Here's the drawing with two shaded views (mm, measured from the low corner). I have some questions. Round coordinates to 2 decimals unless told otherwise and drop trailing zeros. Write each loop counter-clockwise with the first axis right and the second up, starting at its lowest first coordinate (ties: lowest second). Pieces come first, ordered by that corner, then holes. Notation, with made-up numbers: M 8,-29.5 L 22,-29.5 A34 cw 22,8.5 Z; hole C -32.75,17 d10. An arc over 180 degrees is marked long. Answer as a JSON object with one key per item and string values. Group by question number.
1) I'm going to push flat-ended pins straight in: pin 1 Ø2 at (x, z) = (46, 46) entering from -Y; pin 2 Ø3 at (y, z) = (49, 26) entering from -X; pin 3 Ø12 at (x, y) = (67, 35) entering from +Z. Where does each tip first touch, or does it pass through?
2) Suppose I cut it at A-A, the plane x = 50. Write out the boundary of the cut face in (y, z), and give its area (3 significant figures).
3) Suppose I cut it at B-B, the plane y = 48. Write out the boundary of the cut face in (x, z).
4) Suppose I cut it at C-C, the plane z = 24. Write out the boundary of the cut face in (x, y).
5) Suppose I cut it at D-D, the plane x = 92. Write out the boundary of the cut face in (y, z), and give its area (3 significant figures).
6) Please list where these lines run through material, in increasing order: L1, parallel to Z at x = 48.5, y = 43; L2, parallel to Z at x = 50, y = 57; L3, parallel to Y at x = 64, z = 27. Write a range as [from, to].
7) If we mould it in two halves opening along X, with no side actions, what happens to the marked faces 1, 2, 3 and 4? For each: +X half, -X half, draft (parallel to the pull), parting line (faces both ways), or undercut.
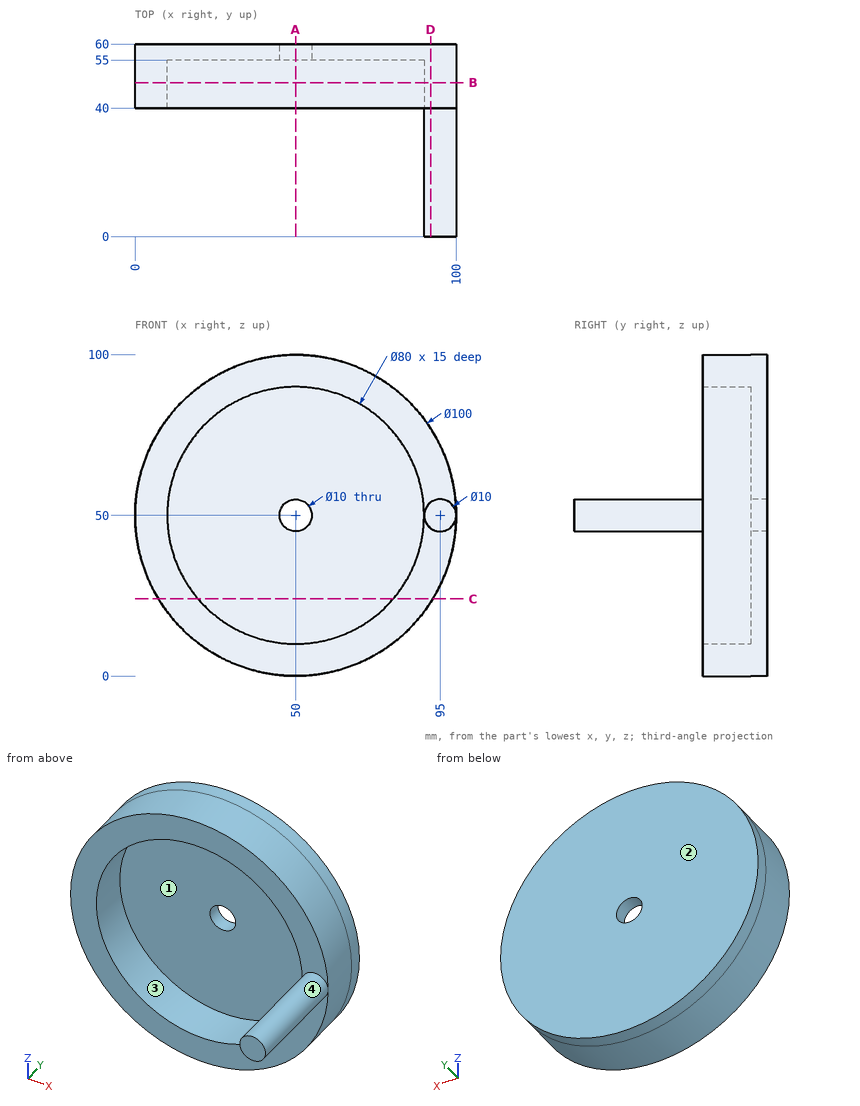
Results:
{
 "1": {"pin 1": "y = 55", "pin 2": "x = 5.35", "pin 3": "z = 98.09"},
 "2": {"outline": "M 40,0 L 60,0 L 60,45 L 55,45 L 55,10 L 40,10 Z; M 40,90 L 55,90 L 55,55 L 60,55 L 60,100 L 40,100 Z", "area": "750 mm^2"},
 "3": {"outline": "C 50,50 d100; hole C 50,50 d80"},
 "4": {"outline": "M 7.29,40 L 19.6,40 L 19.6,55 L 80.4,55 L 80.4,40 L 92.71,40 L 92.71,60 L 7.29,60 Z"},
 "5": {"outline": "M 0,46 L 40,46 L 40,22.87 L 60,22.87 L 60,77.13 L 40,77.13 L 40,54 L 0,54 Z", "area": "1,410 mm^2"},
 "6": {"L1": "[0.02, 10.03], [89.97, 99.98]", "L2": "[0, 45], [55, 100]", "L3": "[55, 60]"},
 "7": {"face 1": "undercut", "face 2": "draft", "face 3": "undercut", "face 4": "parting line"}
}
